The figure shows three views and two pictorial views of one solid part (mm, origin at its lowest corner). Answer the questions. A direction names the side the tool comes from. Give positions to 0.01 mm unless a question says otherwise; leave off trailing zeros. Loops run counter-clockwise (first coordinate to the right, second up) from the corner with the lowest first, then second, coordinate; pieces in that order, holes last. Notation, with made-up numbers: (1.5, 64.25) -> (19.5, 64.25) arc R13 cw to (19.5, 89.25) -> close; hole circle Ø4 at (89, 40). An arc over 180 degrees is marked (long way). One line per item, written item: value. Start each with the question number.
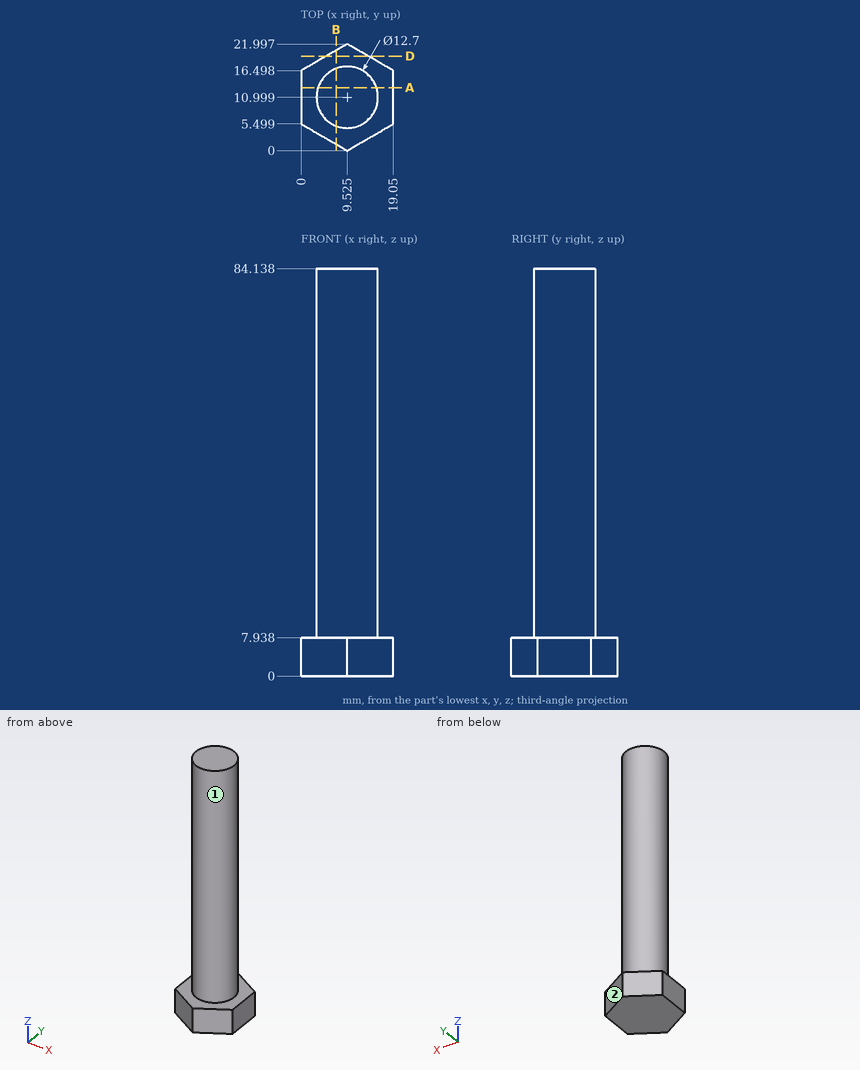
Item 1: For the marked faces 1 and 2, determine the directions among +Z, -Z, +X, -X, +Y, -Y from which every point of the face is accessible in a straight line to the end or side of a thin tool.
Item 2: Flat-ended cylindrical pins translate along their axes: pin 1 (4 mm diameter, centred on x = 7.5, z = 61, fed in from +Y); pin 2 (2 mm diameter, centred on y = 9.5, z = 23.5, fed in from +X) (1 decimal); pin 3 (6 mm diameter, centred on y = 10, z = 33.5, fed in from -X) (1 decimal). Find the tip coordinate at first contact, or state that the pin passes through.
Item 3: Consider L1, parallel to Z at x = 6.75, y = 1.75; L2, parallel to Y at x = 8, z = 21.5 (1 decimal); L3, parallel to X at y = 15.75, z = 70 (1 decimal). Determine where each line is inside the solid, lowest interval first. Write a range as [from, to].
Item 4: Section D-D, the plane y = 19.5 is taken. Determine the outline of the cut face in (x, z).
Item 5: Section B-B, the plane x = 7.25 is taken. Determine the outline of the cut face in (y, z), plus the area to 3 significant figures.
Item 6: Section A-A, the plane y = 13 is taken. Determine the outline of the cut face in (x, z), plus the area to 3 significant figures.
Computed values:
1. face 1: +Z
1. face 2: +Z, -Z, +X, +Y
2. pin 1: y = 17.35
2. pin 2: x = 15.9
2. pin 3: x = 3.2
3. L1: [0, 7.94]
3. L2: [4.8, 17.2]
3. L3: [5.3, 13.7]
4. outline: (5.2, 0) -> (13.85, 0) -> (13.85, 7.94) -> (5.2, 7.94) -> close
5. outline: (1.31, 0) -> (20.68, 0) -> (20.68, 7.94) -> (16.93, 7.94) -> (16.93, 84.14) -> (5.07, 84.14) -> (5.07, 7.94) -> (1.31, 7.94) -> close
5. area: 1,060 mm²
6. outline: (0, 0) -> (19.05, 0) -> (19.05, 7.94) -> (15.55, 7.94) -> (15.55, 84.14) -> (3.5, 84.14) -> (3.5, 7.94) -> (0, 7.94) -> close
6. area: 1,070 mm²
